Can you work these out from the model? Positions are in its coordinate system, mm. Face numbers are marked on the shaded views. Round coordinates to 2 decimals unless told otherwise and drop trailing zeros. Loops run counter-clockwise (first coordinate to the right, second up) from the corner with the lowest first, then second, coordinate; pieces in that order, holes last. Notation, with made-up numbers: (-25, 30) - (-12, 30) arc R9 cw to (-12, 36) - close; hole circle Ø11 at (47.5, 23.5). An arc over 180 degrees is marked (long way). Answer as CSV lines item,"result".
```python
from build123d import *

# Parameters (mm, degrees)
SKETCH1_R           = 1.5
BOSS_EXTRUDE1_DEPTH = 10
CUT_EXTRUDE1_REACH  = 8.5
SKETCH2_R           = 2.6


with BuildPart() as part:
    # Sketch1 → Boss-Extrude1 (new body)
    with BuildSketch(Plane(origin=(0, 0, 0), x_dir=(1, 0, 0), z_dir=(0, 1, 0))):
        with BuildLine():
            Line((0, 0), (12.309647022, 0))
            ThreePointArc((12.309647022, 0), (15.100505063, 1.899494937), (17.891363104, 0))
            Line((17.891363104, 0), (32.108636896, 0))
            ThreePointArc((32.108636896, 0), (34.899494937, 1.899494937), (37.690352978, 0))
            Line((37.690352978, 0), (50, 0))
            Line((50, 0), (50, 6.5))
            Line((50, 6.5), (0, 6.5))
            Line((0, 6.5), (0, 0))
        make_face()
        with Locations((10.5, 3.5)):
            Circle(SKETCH1_R, mode=Mode.SUBTRACT)
        with Locations((39.5, 3.5)):
            Circle(SKETCH1_R, mode=Mode.SUBTRACT)
    extrude(amount=BOSS_EXTRUDE1_DEPTH)

    # Sketch2 → Cut-Extrude1 (cut, up to next)
    with BuildSketch(Plane.XY, mode=Mode.PRIVATE) as cut_extrude1_sk1:
        with Locations((5, 5)):
            Circle(SKETCH2_R)
    cut_extrude1_tool1 = extrude(cut_extrude1_sk1.sketch, amount=-CUT_EXTRUDE1_REACH, mode=Mode.PRIVATE) & part.part
    add(cut_extrude1_tool1.solids().sort_by_distance((5, 5, 0))[0], mode=Mode.SUBTRACT)
    # Sketch2 → Cut-Extrude1 (cut, up to next)
    with BuildSketch(Plane.XY, mode=Mode.PRIVATE) as cut_extrude1_sk2:
        with Locations((45, 5)):
            Circle(SKETCH2_R)
    cut_extrude1_tool2 = extrude(cut_extrude1_sk2.sketch, amount=-CUT_EXTRUDE1_REACH, mode=Mode.PRIVATE) & part.part
    add(cut_extrude1_tool2.solids().sort_by_distance((45, 5, 0))[0], mode=Mode.SUBTRACT)


solid = part.part
```
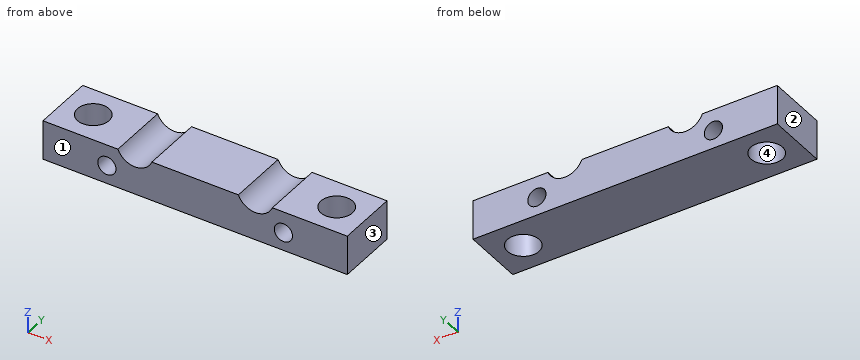
Q1. I'm going to push flat-ended pins straight in: pin 1 Ø1 at (x, z) = (38, -2) entering from -Y; pin 2 Ø4.5 at (x, y) = (45, 5) entering from +Z. Where does each tip first touch, or does it pass through?
Checks:
pin 1,"y = 0"
pin 2,"through"
Q2. If I drill on line 1 along X through (y, z) = (1, -3.5); line 2 along X through (y, z) = (2, -4.5); line 3 along Z through (x, y) = (39.5, 3.5), over which ranges is the centre line in solid material (lowest first)? Write a range as [from, to].
Checks:
line 1,"[0, 9], [12, 38], [41, 50]"
line 2,"[0, 9.38], [11.62, 38.38], [40.62, 50]"
line 3,"[-6.5, -5], [-2, 0]"
Q3. We'd pull the mould along X, two halves only. Please class the marked faces 1, 2, 3 and 4: pulls with the +X half, pulls with the -X half, needs draft (parallel to the pull), parting line crosses it, or undercut.
Checks:
face 1,"needs draft"
face 2,"pulls with the -X half"
face 3,"pulls with the +X half"
face 4,"undercut"
Q4. Imagine slicing it at D-D (y = 1). Write out the boundary of the cut face in (x, z).
Checks:
outline,"(0, -6.5) - (50, -6.5) - (50, 0) - (37.69, 0) arc R3 cw to (32.11, 0) - (17.89, 0) arc R3 cw to (12.31, 0) - (0, 0) - close; hole circle Ø3 at (10.5, -3.5); hole circle Ø3 at (39.5, -3.5)"
Q5. Imagine slicing it at A-A (y = 4). Write out the boundary of the cut face in (x, z), then the cut area to 3 significant figures.
Checks:
outline,"(0, -6.5) - (2.6, -6.5) - (2.6, 0) - (0, 0) - close; (7.4, -6.5) - (42.6, -6.5) - (42.6, 0) - (37.69, 0) arc R3 cw to (32.11, 0) - (17.89, 0) arc R3 cw to (12.31, 0) - (7.4, 0) - close; (47.4, -6.5) - (50, -6.5) - (50, 0) - (47.4, 0) - close; hole circle Ø3 at (10.5, -3.5); hole circle Ø3 at (39.5, -3.5)"
area,"233 mm²"
Q6. Imagine slicing it at C-C (x = 5). Write out the boundary of the cut face in (y, z).
Checks:
outline,"(0, -6.5) - (2.4, -6.5) - (2.4, 0) - (0, 0) - close; (7.6, -6.5) - (10, -6.5) - (10, 0) - (7.6, 0) - close"
Q7. Imagine slicing it at B-B (z = -3.5). Write out the boundary of the cut face in (x, y).
Checks:
outline,"(0, 0) - (9, 0) - (9, 10) - (0, 10) - close; (12, 0) - (38, 0) - (38, 10) - (12, 10) - close; (41, 0) - (50, 0) - (50, 10) - (41, 10) - close; hole circle Ø5.2 at (5, 5); hole circle Ø5.2 at (45, 5)"
